Design review of the part built by this model. Coordinates are the model's own, in mm. Coordinates: 2 decimals unless noted, no trailing zeros. Write each loop counter-clockwise with the first axis right and the second up, starting at its lowest first coordinate (ties: lowest second). Pieces come first, ordered by that corner, then holes. Notation, with made-up numbers: M 66,-38 L 98,-38 A19 cw 98,-6 Z; hole C 36,74.25 d2. An arc over 180 degrees is marked long. Write item = value, one per line.
Autodesk Inventor part; units mm, degrees
ref_plane "YZ Plane" through (0, 0, 0) normal (1, 0, 0) x (0, 1, 0)
ref_plane "XZ Plane" through (0, 0, 0) normal (0, 1, 0) x (-1, 0, 0)
ref_plane "XY Plane" through (0, 0, 0) normal (0, 0, 1) x (1, 0, 0)
sketch "Sketch1" plane through (0, 0, 0) normal (0, 1, 0) x (-1, 0, 0)
  circle A0 centre (0, 0) radius 6
  dimension "d0" = 12
extrude "Extrusion1" add sketch "Sketch1" along normal blind 800
sketch "Sketch2" plane through (0, 800, 0) normal (0, 1, 0) x (1, 0, 0)
  circle A0 centre (0, 0) radius 6
hole "Hole1" at (0, 800, 0) direction (0, -1, 0) diameter 8 depth 33 tip angle 118
sketch "Sketch3" plane through (0, 0, 0) normal (0, -1, 0) x (1, 0, 0)
  circle A0 centre (0, 0) radius 6
hole "Hole2" at (0, 0, 0) direction (0, 1, 0) diameter 8 depth 33 tip angle 118
sketch "Sketch5" plane through (0, 0, 0) normal (0, 0, 1) x (1, 0, 0)
  line L0 (-6, 0) -> (-6, 800)
  line L1 (6, 0) -> (6, 800)
  line L2 (-4, 800) -> (4, 800)
  line L3 (4, 0) -> (-4, 0)
  line L4 (0, 0) -> (0, 800)
  circle A0 centre (0, 400) radius 2
  dimension "d22" = 4
extrude "Extrusion3" cut sketch "Sketch5" against normal through all both and the other way through all
thread "Thread2"
properties part number "lower arm 800"
Q1. For P1, Ø1, axis at y = 663.5, z = 3.5, coming from the -X side, flat-tipped, find the tip position at first contact; note if it passes through.
Check result:
P1 = -5.2
Q2. Wall thickness on line 1 (X direction, y = 400, z = -0.25); line 2 (Z direction, x = 0, y = 13.5); line 3 (X direction, y = 447.5, z = 0.25): over which ranges is each line inside the solid? List them lowest first.
Check result:
line_1 = -5.99 to -2, 2 to 5.99
line_2 = -6 to -4, 4 to 6
line_3 = -5.99 to 5.99
Q3. Consider section A-A, the plane y = 733.5. State the section outline as (x, z) points, and give its area (3 significant figures).
Check result:
outline = C 0,0 d12
area = 113 mm²
